Read the model definition and answer for the solid it produces. Units are mm, in the model's axes. Face numbers are marked on the shaded views. A direction names the side the tool comes from. Coordinates: 2 decimals unless noted, no trailing zeros. Write each loop counter-clockwise with the first axis right and the second up, starting at its lowest first coordinate (ties: lowest second). Pieces come first, ordered by that corner, then holes.
1) The part is cut by section A-A (x = 0.5). Determine the outline of the cut face in (y, z) (3 decimals), then the cut area to 3 significant figures.
2) The part is cut by section B-B (z = 0). Determine the outline of the cut face in (x, y) (3 decimals), then the cut area to 3 significant figures.
3) Find the intervals of material crossed by line 1 (Y direction, x = 1.5, z = -0.05); line 2 (X direction, y = -1.3, z = -0.45); line 3 (Z direction, x = 4.75, y = -1.8), in increasing order.
4) The part is cut by section D-D (x = -7.25). Determine the outline of the cut face in (y, z) (3 decimals), then the cut area to 3 significant figures.
5) The part is cut by section C-C (y = -1.75). Determine the outline of the cut face in (x, z), then the cut area to 3 significant figures.
6) Determine the mould class of the marked faces 3, 4, 5 and 6 for opening direction Z: +Z half, -Z half, draft (parallel to the pull), parting line (faces both ways), or undercut.
7) Each of these flat-tipped pins is pushed along its axis until it touches: pin 1 Ø0.8 at (x, z) = (1.5, -0.5) entering from -Y; pin 2 Ø1 at (x, z) = (3.5, -1) entering from -Y. Where does it stop, or does it pass through?
8) Which of the six approach directions +Z, -Z, +X, -X, +Y, -Y give full straight-line access (tool end or side, diameter ignored) to the marked faces 1 and 2?
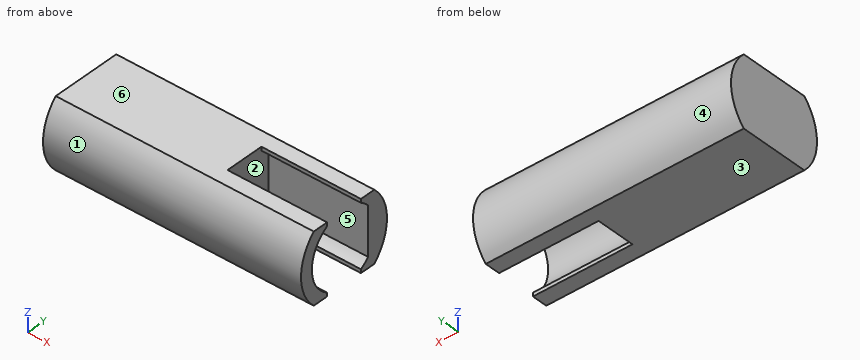
from build123d import *

# Parameters (mm, degrees)
BOSS_EXTRUDE1_DEPTH   = 5.4
BOSS_EXTRUDE1_2_DEPTH = 5.4
BOSS_EXTRUDE2_START   = 8.6
BOSS_EXTRUDE2_DEPTH   = 8.6


with BuildPart() as part:
    # Sketch2 → Boss-Extrude1 (new body)
    with BuildSketch(Plane(origin=(0, 0, 0), x_dir=(0, 0, -1), z_dir=(1, 0, 0))):
        with BuildLine():
            Line((-1.9, -1.882983006), (-1.9, -1.053565375))
            Line((-1.9, -1.053565375), (-1.7, -1.053565375))
            ThreePointArc((-1.7, -1.053565375), (0, -2), (1.7, -1.053565375))
            Line((1.7, -1.053565375), (1.9, -1.053565375))
            Line((1.9, -1.053565375), (1.9, -1.882983006))
            ThreePointArc((1.9, -1.882983006), (0, -2.675), (-1.9, -1.882983006))
        make_face()
    extrude(amount=BOSS_EXTRUDE1_DEPTH)



with BuildPart() as body_2:
    # Sketch2 → Boss-Extrude1 2 (new body)
    with BuildSketch(Plane(origin=(0, 0, 0), x_dir=(0, 0, -1), z_dir=(1, 0, 0))):
        with BuildLine():
            Line((-1.9, 1.882983006), (-1.9, 1.053565375))
            Line((-1.9, 1.053565375), (-1.7, 1.053565375))
            ThreePointArc((-1.7, 1.053565375), (-1.527831887, 1.290631521), (-1.322875656, 1.5))
            Line((-1.322875656, 1.5), (1.322875656, 1.5))
            ThreePointArc((1.322875656, 1.5), (1.527831887, 1.290631521), (1.7, 1.053565375))
            Line((1.7, 1.053565375), (1.9, 1.053565375))
            Line((1.9, 1.053565375), (1.9, 1.882983006))
            ThreePointArc((1.9, 1.882983006), (0, 2.675), (-1.9, 1.882983006))
        make_face()
    extrude(amount=BOSS_EXTRUDE1_2_DEPTH)


with BuildPart() as part_1:
    add(part.part)

    add(body_2.part)  # Boss-Extrude2 merges body 2
    # Sketch3 → Boss-Extrude2 (add)
    with BuildSketch(Plane.ZY.offset(BOSS_EXTRUDE2_START)):
        with BuildLine():
            Line((1.9, -1.882983006), (1.9, 1.882983006))
            ThreePointArc((1.9, 1.882983006), (0, 2.675), (-1.9, 1.882983006))
            Line((-1.9, 1.882983006), (-1.9, -1.882983006))
            ThreePointArc((-1.9, -1.882983006), (0, -2.675), (1.9, -1.882983006))
        make_face()
    extrude(amount=-BOSS_EXTRUDE2_DEPTH)


solid = part_1.part
Reported:
1. outline: (-1.883, -1.9) - (-1.054, -1.9) - (-1.054, -1.7) arc R2 cw to (-1.054, 1.7) - (-1.054, 1.9) - (-1.883, 1.9) arc R2.675 ccw to start; (1.054, -1.9) - (1.883, -1.9) arc R2.675 ccw to (1.883, 1.9) - (1.054, 1.9) - (1.054, 1.7) arc R2 cw to (1.5, 1.323) - (1.5, -1.323) arc R2 cw to (1.054, -1.7) - close
1. area: 6.81 mm2
2. outline: (-8.6, -2.675) - (5.4, -2.675) - (5.4, -2) - (0, -2) - (0, 1.5) - (5.4, 1.5) - (5.4, 2.675) - (-8.6, 2.675) - close
2. area: 56.0 mm2
3. line 1: y = -2.67 to -2, 1.5 to 2.67
3. line 2: x = -8.6 to 0
3. line 3: z = -1.9 to -0.87, 0.87 to 1.9
4. outline: (-1.883, -1.9) - (1.883, -1.9) arc R2.675 ccw to (1.883, 1.9) - (-1.883, 1.9) arc R2.675 ccw to start
4. area: 18.5 mm2
5. outline: (-8.6, -1.9) - (5.4, -1.9) - (5.4, -0.97) - (0, -0.97) - (0, 0.97) - (5.4, 0.97) - (5.4, 1.9) - (-8.6, 1.9) - close
5. area: 42.7 mm2
6. face 3: -Z half
6. face 4: parting line
6. face 5: undercut
6. face 6: +Z half
7. pin 1: stops at y = -2.67
7. pin 2: stops at y = -2.63
8. face 1: +X, -X, -Y
8. face 2: +X
